Input: dimensioned drawing with shaded views. Units: mm. Origin: part minimum x, y, z. Round coordinates to 2 decimals unless told otherwise and drop trailing zeros. Write each loop counter-clockwise with the first axis right and the second up, starting at its lowest first coordinate (ties: lowest second). Pieces come first, ordered by that corner, then holes. Notation, with made-up numbers: M 83,78.5 L 92,78.5 A27 cw 92,107.5 Z; hole C 34,33 d10. An arc over 180 degrees is marked long. Use one line per item in the form item = value. Start each with the question number.
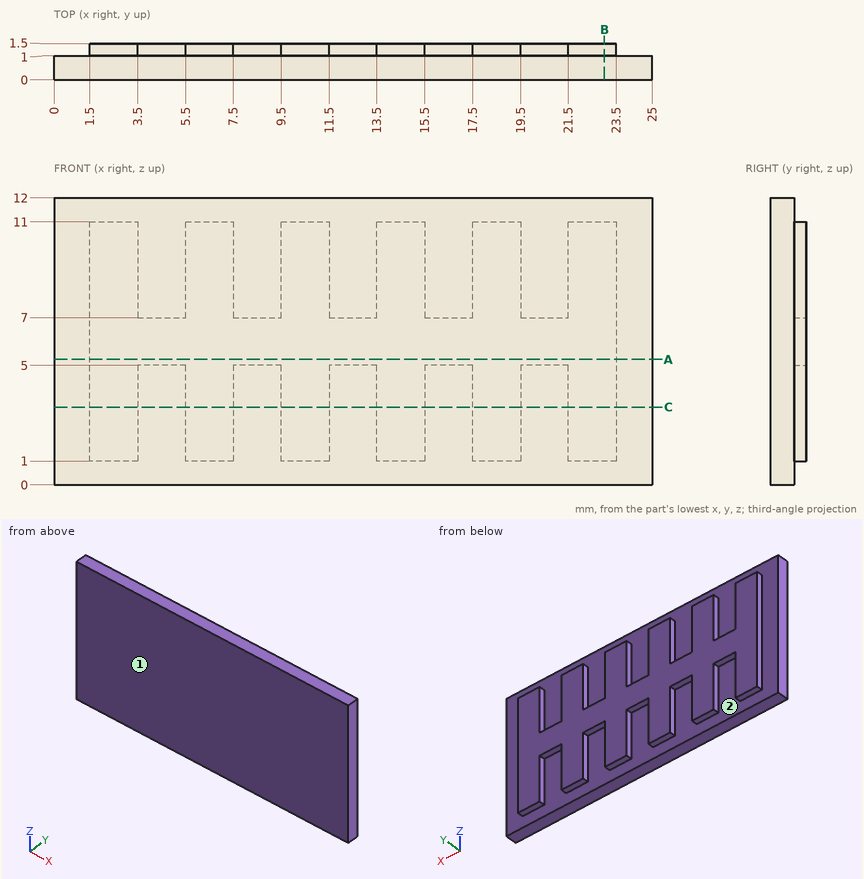
1. Ray query, probe 1 along X at (y, z) = (1.1, 10.25); probe 2 along Y at (x, z) = (1.25, 7.5); probe 3 along X at (y, z) = (1.3, 6.25). Return the intervals inside material, ascending.
2. Pull-direction query (X, two-part tool) for the marked faces 1 and 2; classes: released by +X, released by -X, zero draft, split by the parting line, or undercut.
3. Section query A-A (z = 5.25). Return loops of the section in (x, y), then the cut area to 3 significant figures.
4. Section query C-C (z = 3.25). Return loops of the section in (x, y), then the cut area to 3 significant figures.
5. Section query B-B (x = 23). Return loops of the section in (y, z), then the cut area to 3 significant figures.
6. Contact query for flat-ended pins moving along their axis: pin 1 (0.6 mm diameter, centred on x = 20.5, y = 1.5, fed in from +Z); pin 2 (1 mm diameter, centred on x = 13, z = 10.5, fed in from -Y); pin 3 (0.6 mm diameter, centred on x = 16.5, y = 1.5, fed in from -Z). Output: stop coordinate, or through.
Checks:
q1.probe_1 = 1.5 to 3.5, 5.5 to 7.5, 9.5 to 11.5, 13.5 to 15.5, 17.5 to 19.5, 21.5 to 23.5
q1.probe_2 = 0 to 1
q1.probe_3 = 1.5 to 23.5
q2.face_1 = zero draft
q2.face_2 = undercut
q3.outline = M 0,0 L 25,0 L 25,1 L 23.5,1 L 23.5,1.5 L 1.5,1.5 L 1.5,1 L 0,1 Z
q3.area = 36.0 mm^2
q4.outline = M 0,0 L 25,0 L 25,1 L 23.5,1 L 23.5,1.5 L 21.5,1.5 L 21.5,1 L 19.5,1 L 19.5,1.5 L 17.5,1.5 L 17.5,1 L 15.5,1 L 15.5,1.5 L 13.5,1.5 L 13.5,1 L 11.5,1 L 11.5,1.5 L 9.5,1.5 L 9.5,1 L 7.5,1 L 7.5,1.5 L 5.5,1.5 L 5.5,1 L 3.5,1 L 3.5,1.5 L 1.5,1.5 L 1.5,1 L 0,1 Z
q4.area = 31.0 mm^2
q5.outline = M 0,0 L 1,0 L 1,1 L 1.5,1 L 1.5,11 L 1,11 L 1,12 L 0,12 Z
q5.area = 17.0 mm^2
q6.pin_1 = 7
q6.pin_2 = 0
q6.pin_3 = 5
